```python
from build123d import *

# Parameters (mm, degrees)
SKETCH1_W                        = 170
SKETCH1_H                        = 150
BOSS_EXTRUDE1_DEPTH              = 5
FILLET1_R                        = 10
BOSS_EXTRUDE2_DEPTH              = 38
SKETCH29_W                       = 43
SKETCH29_H                       = 5
BOSS_EXTRUDE3_DEPTH              = 19
CUT_EXTRUDE1_START               = -2.9
SKETCH6_R                        = 16.5
CUT_EXTRUDE1_DEPTH               = 93.9
SKETCH13_R                       = 5.1
CUT_EXTRUDE2_DEPTH               = 4.7
TAP_DRILL_FOR_M2_TAP1_AT_2_COUNT = 2
TAP_DRILL_FOR_M2_TAP1_AT_2_PITCH = 8.5
TAP_DRILL_FOR_M2_TAP1_AT_3_COUNT = 2
TAP_DRILL_FOR_M2_TAP1_AT_3_PITCH = 14.722431864
TAP_DRILL_FOR_M2_TAP1_AT_4_COUNT = 2
TAP_DRILL_FOR_M2_TAP1_AT_4_PITCH = 14.722431864
FILLET2_R                        = 5
SKETCH28_W                       = 33
SKETCH28_H                       = 20
CUT_EXTRUDE3_DEPTH               = 10
MIRROR25_COPY_4_DEPTH            = 38
MIRROR25_START                   = -2.9
MIRROR25_COPY_5_SKETCH_R         = 16.5
MIRROR25_COPY_5_DEPTH            = 93.9
MIRROR25_COPY_6_SKETCH_R         = 5.1
MIRROR25_COPY_6_DEPTH            = 4.7
MIRROR25_COPY_11_SKETCH_W        = 33
MIRROR25_COPY_11_SKETCH_H        = 20
MIRROR25_COPY_11_DEPTH           = 10
FILLET4_R                        = 5
SKETCH33_W                       = 5
SKETCH33_H                       = 5.425553346
CUT_EXTRUDE4_DEPTH               = 10
CUT_EXTRUDE5_START               = -11
SKETCH34_W                       = 5
SKETCH34_H                       = 5
CUT_EXTRUDE5_DEPTH               = 28
MIRROR29_COPY_1_SKETCH_W         = 43
MIRROR29_COPY_1_SKETCH_H         = 5
MIRROR29_COPY_1_DEPTH            = 19
MIRROR29_START                   = -2.9
MIRROR29_COPY_2_SKETCH_R         = 16.5
MIRROR29_COPY_2_DEPTH            = 93.9
MIRROR29_COPY_3_SKETCH_W         = 5
MIRROR29_COPY_3_SKETCH_H         = 5.425553346
MIRROR29_COPY_3_DEPTH            = 10
MIRROR29_START_2                 = -11
MIRROR29_COPY_4_SKETCH_W         = 5
MIRROR29_COPY_4_SKETCH_H         = 5
MIRROR29_COPY_4_DEPTH            = 28


with BuildPart() as part:
    # Sketch1 → Boss-Extrude1 (new body)
    with BuildSketch(Plane(origin=(0, 0, 0), x_dir=(1, 0, 0), z_dir=(0, 1, 0))):
        Rectangle(SKETCH1_W, SKETCH1_H)
    extrude(amount=BOSS_EXTRUDE1_DEPTH)

    # Fillet1
    fillet1_edges = [part.edges().sort_by_distance(p)[0] for p in [
        (85, 2.5, 75),
        (-85, 2.5, 75),
        (-85, 2.5, -75),
        (85, 2.5, -75),
    ]]
    fillet(fillet1_edges, radius=FILLET1_R)

    # Sketch3 → Boss-Extrude2 (add)
    with BuildSketch(Plane.XZ):
        Polygon((-75, 75), (-75, 60), (-70, 60), (-70, 70), (-37, 70), (-37, 60), (-32, 60), (-32, 75), align=None)
    boss_extrude2 = extrude(amount=BOSS_EXTRUDE2_DEPTH)

    # Sketch29 → Boss-Extrude3 (add)
    with BuildSketch(Plane.XZ):
        with Locations((-53.5, 36.727703087)):
            Rectangle(SKETCH29_W, SKETCH29_H)
    boss_extrude3 = extrude(amount=BOSS_EXTRUDE3_DEPTH)

    # Sketch6 → Cut-Extrude1 (cut)
    with BuildSketch(Plane(origin=(0, 0, 70), x_dir=(-1, 0, 0), z_dir=(0, 0, -1)).offset(CUT_EXTRUDE1_START)):
        with Locations((53.5, -19)):
            Circle(SKETCH6_R)
    cut_extrude1 = extrude(amount=CUT_EXTRUDE1_DEPTH, mode=Mode.SUBTRACT)

    # Sketch13 → Cut-Extrude2 (cut)
    with BuildSketch(Plane(origin=(0, 0, 72.9), x_dir=(-1, 0, 0), z_dir=(0, 0, -1))):
        with Locations((53.5, -19)):
            Circle(SKETCH13_R)
    cut_extrude2 = extrude(amount=-CUT_EXTRUDE2_DEPTH, mode=Mode.SUBTRACT)

    # Sketch16 → Tap Drill for M2 Tap1 (revolve, cut)
    with BuildSketch(Plane(origin=(-46.138784068, -23.25, 72.9), x_dir=(0, 1, 0), z_dir=(1, 0, 0))):
        Polygon((0, 0), (0, 4.080688495), (0.8, 3.6), (0.8, 0), align=None)
    tap_drill_for_m2_tap1 = revolve(axis=Axis((-46.138784068, -23.25, 66.55), (0, 0, 1)), mode=Mode.SUBTRACT)

    # Tap Drill for M2 Tap1 at 2: Tap Drill for M2 Tap1 ×2
    with Locations(*[Vector(-0.86602540378444, -0.49999999999999756, 0) * (i * TAP_DRILL_FOR_M2_TAP1_AT_2_PITCH) for i in range(1, TAP_DRILL_FOR_M2_TAP1_AT_2_COUNT)]):
        add(tap_drill_for_m2_tap1, mode=Mode.SUBTRACT)

    # Tap Drill for M2 Tap1 at 3: Tap Drill for M2 Tap1 ×2
    with Locations(*[(-i * TAP_DRILL_FOR_M2_TAP1_AT_3_PITCH, 0, 0) for i in range(1, TAP_DRILL_FOR_M2_TAP1_AT_3_COUNT)]):
        add(tap_drill_for_m2_tap1, mode=Mode.SUBTRACT)

    # Tap Drill for M2 Tap1 at 4: Tap Drill for M2 Tap1 ×2
    with Locations(*[Vector(-0.49999999999999784, 0.8660254037844399, 0) * (i * TAP_DRILL_FOR_M2_TAP1_AT_4_PITCH) for i in range(1, TAP_DRILL_FOR_M2_TAP1_AT_4_COUNT)]):
        add(tap_drill_for_m2_tap1, mode=Mode.SUBTRACT)

    # Fillet2
    fillet2_edges = [part.edges().sort_by_distance(p)[0] for p in [
        (-32, -19, 75),
        (-75, -19, 75),
    ]]
    fillet(fillet2_edges, radius=FILLET2_R)

    # Sketch28 → Cut-Extrude3 (cut)
    with BuildSketch(Plane.XZ):
        with Locations((-53.5, 16.617641144)):
            Rectangle(SKETCH28_W, SKETCH28_H)
    cut_extrude3 = extrude(amount=-CUT_EXTRUDE3_DEPTH, mode=Mode.SUBTRACT)

    # Mirror14: Boss-Extrude2 across plane
    add(boss_extrude2.mirror(Plane.XY))

    # Mirror15: Cut-Extrude1, Cut-Extrude2 across plane
    add(cut_extrude1.mirror(Plane.XY), mode=Mode.SUBTRACT)
    add(cut_extrude2.mirror(Plane.XY), mode=Mode.SUBTRACT)

    # Mirror16: Tap Drill for M2 Tap1 across plane
    add(tap_drill_for_m2_tap1.mirror(Plane.XY), mode=Mode.SUBTRACT)

    # Mirror16 copy 1 sketch → Mirror16 copy 1 (revolve, cut)
    with BuildSketch(Plane(origin=(-53.5, -27.5, -72.9), x_dir=(0, 1, 0), z_dir=(1, 0, 0))):
        Polygon((0, 0), (0, -4.080688495), (0.8, -3.6), (0.8, 0), align=None)
    revolve(axis=Axis((-53.5, -27.5, -66.55), (0, 0, 1)), mode=Mode.SUBTRACT)

    # Mirror16 copy 2 sketch → Mirror16 copy 2 (revolve, cut)
    with BuildSketch(Plane(origin=(-60.861215932, -23.25, -72.9), x_dir=(0, 1, 0), z_dir=(1, 0, 0))):
        Polygon((0, 0), (0, -4.080688495), (0.8, -3.6), (0.8, 0), align=None)
    revolve(axis=Axis((-60.861215932, -23.25, -66.55), (0, 0, 1)), mode=Mode.SUBTRACT)

    # Mirror16 copy 3 sketch → Mirror16 copy 3 (revolve, cut)
    with BuildSketch(Plane(origin=(-53.5, -10.5, -72.9), x_dir=(0, 1, 0), z_dir=(1, 0, 0))):
        Polygon((0, 0), (0, -4.080688495), (0.8, -3.6), (0.8, 0), align=None)
    revolve(axis=Axis((-53.5, -10.5, -66.55), (0, 0, 1)), mode=Mode.SUBTRACT)

    # Mirror24: Cut-Extrude3 across plane
    add(cut_extrude3.mirror(Plane.XY), mode=Mode.SUBTRACT)

    # Mirror25: Boss-Extrude2, Cut-Extrude1, Cut-Extrude2, Tap Drill for M2 Tap1, Cut-Extrude3 across plane
    add(boss_extrude2.mirror(Plane(origin=(0, 0, 0), x_dir=(0, 0, 1), z_dir=(1, 0, 0))))
    add(cut_extrude1.mirror(Plane(origin=(0, 0, 0), x_dir=(0, 0, 1), z_dir=(1, 0, 0))), mode=Mode.SUBTRACT)
    add(cut_extrude2.mirror(Plane(origin=(0, 0, 0), x_dir=(0, 0, 1), z_dir=(1, 0, 0))), mode=Mode.SUBTRACT)
    add(tap_drill_for_m2_tap1.mirror(Plane(origin=(0, 0, 0), x_dir=(0, 0, 1), z_dir=(1, 0, 0))), mode=Mode.SUBTRACT)
    add(cut_extrude3.mirror(Plane(origin=(0, 0, 0), x_dir=(0, 0, 1), z_dir=(1, 0, 0))), mode=Mode.SUBTRACT)

    # Mirror25 copy 1 sketch → Mirror25 copy 1 (revolve, cut)
    with BuildSketch(Plane(origin=(53.5, -27.5, 72.9), x_dir=(0, 1, 0), z_dir=(-1, 0, 0))):
        Polygon((0, 0), (0, -4.080688495), (0.8, -3.6), (0.8, 0), align=None)
    revolve(axis=Axis((53.5, -27.5, 66.55), (0, 0, -1)), mode=Mode.SUBTRACT)

    # Mirror25 copy 2 sketch → Mirror25 copy 2 (revolve, cut)
    with BuildSketch(Plane(origin=(60.861215932, -23.25, 72.9), x_dir=(0, 1, 0), z_dir=(-1, 0, 0))):
        Polygon((0, 0), (0, -4.080688495), (0.8, -3.6), (0.8, 0), align=None)
    revolve(axis=Axis((60.861215932, -23.25, 66.55), (0, 0, -1)), mode=Mode.SUBTRACT)

    # Mirror25 copy 3 sketch → Mirror25 copy 3 (revolve, cut)
    with BuildSketch(Plane(origin=(53.5, -10.5, 72.9), x_dir=(0, 1, 0), z_dir=(-1, 0, 0))):
        Polygon((0, 0), (0, -4.080688495), (0.8, -3.6), (0.8, 0), align=None)
    revolve(axis=Axis((53.5, -10.5, 66.55), (0, 0, -1)), mode=Mode.SUBTRACT)

    # Mirror25 copy 4 sketch → Mirror25 copy 4 (add)
    with BuildSketch(Plane(origin=(0, 0, 0), x_dir=(-1, 0, 0), z_dir=(0, -1, 0))):
        Polygon((-75, 75), (-75, 60), (-70, 60), (-70, 70), (-37, 70), (-37, 60), (-32, 60), (-32, 75), align=None)
    extrude(amount=MIRROR25_COPY_4_DEPTH)

    # Mirror25 copy 5 sketch → Mirror25 copy 5 (cut)
    with BuildSketch(Plane.XY.offset(-70).offset(MIRROR25_START)):
        with Locations((53.5, -19)):
            Circle(MIRROR25_COPY_5_SKETCH_R)
    extrude(amount=MIRROR25_COPY_5_DEPTH, mode=Mode.SUBTRACT)

    # Mirror25 copy 6 sketch → Mirror25 copy 6 (cut)
    with BuildSketch(Plane.XY.offset(-72.9)):
        with Locations((53.5, -19)):
            Circle(MIRROR25_COPY_6_SKETCH_R)
    extrude(amount=-MIRROR25_COPY_6_DEPTH, mode=Mode.SUBTRACT)

    # Mirror25 copy 7 sketch → Mirror25 copy 7 (revolve, cut)
    with BuildSketch(Plane(origin=(46.138784068, -23.25, -72.9), x_dir=(0, 1, 0), z_dir=(-1, 0, 0))):
        Polygon((0, 0), (0, 4.080688495), (0.8, 3.6), (0.8, 0), align=None)
    revolve(axis=Axis((46.138784068, -23.25, -66.55), (0, 0, -1)), mode=Mode.SUBTRACT)

    # Mirror25 copy 8 sketch → Mirror25 copy 8 (revolve, cut)
    with BuildSketch(Plane(origin=(53.5, -27.5, -72.9), x_dir=(0, 1, 0), z_dir=(-1, 0, 0))):
        Polygon((0, 0), (0, 4.080688495), (0.8, 3.6), (0.8, 0), align=None)
    revolve(axis=Axis((53.5, -27.5, -66.55), (0, 0, -1)), mode=Mode.SUBTRACT)

    # Mirror25 copy 9 sketch → Mirror25 copy 9 (revolve, cut)
    with BuildSketch(Plane(origin=(60.861215932, -23.25, -72.9), x_dir=(0, 1, 0), z_dir=(-1, 0, 0))):
        Polygon((0, 0), (0, 4.080688495), (0.8, 3.6), (0.8, 0), align=None)
    revolve(axis=Axis((60.861215932, -23.25, -66.55), (0, 0, -1)), mode=Mode.SUBTRACT)

    # Mirror25 copy 10 sketch → Mirror25 copy 10 (revolve, cut)
    with BuildSketch(Plane(origin=(53.5, -10.5, -72.9), x_dir=(0, 1, 0), z_dir=(-1, 0, 0))):
        Polygon((0, 0), (0, 4.080688495), (0.8, 3.6), (0.8, 0), align=None)
    revolve(axis=Axis((53.5, -10.5, -66.55), (0, 0, -1)), mode=Mode.SUBTRACT)

    # Mirror25 copy 11 sketch → Mirror25 copy 11 (cut)
    with BuildSketch(Plane(origin=(0, 0, 0), x_dir=(-1, 0, 0), z_dir=(0, -1, 0))):
        with Locations((-53.5, 16.617641144)):
            Rectangle(MIRROR25_COPY_11_SKETCH_W, MIRROR25_COPY_11_SKETCH_H)
    extrude(amount=-MIRROR25_COPY_11_DEPTH, mode=Mode.SUBTRACT)

    # Fillet4
    fillet4_edges = [part.edges().sort_by_distance(p)[0] for p in [
        (-75, -19, -75),
        (-32, -19, -75),
        (32, -19, -75),
        (75, -19, -75),
        (75, -19, 75),
        (32, -19, 75),
    ]]
    fillet(fillet4_edges, radius=FILLET4_R)

    # Sketch33 → Cut-Extrude4 (cut)
    with BuildSketch(Plane.XZ):
        with Locations((-26.5, 36.94047976)):
            Rectangle(SKETCH33_W, SKETCH33_H)
    cut_extrude4 = extrude(amount=-CUT_EXTRUDE4_DEPTH, mode=Mode.SUBTRACT)

    # Sketch34 → Cut-Extrude5 (cut)
    with BuildSketch(Plane(origin=(0, 5, 0), x_dir=(1, 0, 0), z_dir=(0, 1, 0)).offset(CUT_EXTRUDE5_START)):
        with Locations((-80.5, -36.727703087)):
            Rectangle(SKETCH34_W, SKETCH34_H)
    cut_extrude5 = extrude(amount=CUT_EXTRUDE5_DEPTH, mode=Mode.SUBTRACT)

    # Mirror28: Boss-Extrude3, Cut-Extrude1, Cut-Extrude4, Cut-Extrude5 across plane
    add(boss_extrude3.mirror(Plane.XY))
    add(cut_extrude1.mirror(Plane.XY), mode=Mode.SUBTRACT)
    add(cut_extrude4.mirror(Plane.XY), mode=Mode.SUBTRACT)
    add(cut_extrude5.mirror(Plane.XY), mode=Mode.SUBTRACT)

    # Mirror29: Boss-Extrude3, Cut-Extrude1, Cut-Extrude4, Cut-Extrude5 across plane
    add(boss_extrude3.mirror(Plane(origin=(0, 0, 0), x_dir=(0, 0, 1), z_dir=(1, 0, 0))))
    add(cut_extrude1.mirror(Plane(origin=(0, 0, 0), x_dir=(0, 0, 1), z_dir=(1, 0, 0))), mode=Mode.SUBTRACT)
    add(cut_extrude4.mirror(Plane(origin=(0, 0, 0), x_dir=(0, 0, 1), z_dir=(1, 0, 0))), mode=Mode.SUBTRACT)
    add(cut_extrude5.mirror(Plane(origin=(0, 0, 0), x_dir=(0, 0, 1), z_dir=(1, 0, 0))), mode=Mode.SUBTRACT)

    # Mirror29 copy 1 sketch → Mirror29 copy 1 (add)
    with BuildSketch(Plane(origin=(0, 0, 0), x_dir=(-1, 0, 0), z_dir=(0, -1, 0))):
        with Locations((-53.5, 36.727703087)):
            Rectangle(MIRROR29_COPY_1_SKETCH_W, MIRROR29_COPY_1_SKETCH_H)
    extrude(amount=MIRROR29_COPY_1_DEPTH)

    # Mirror29 copy 2 sketch → Mirror29 copy 2 (cut)
    with BuildSketch(Plane.XY.offset(-70).offset(MIRROR29_START)):
        with Locations((53.5, -19)):
            Circle(MIRROR29_COPY_2_SKETCH_R)
    extrude(amount=MIRROR29_COPY_2_DEPTH, mode=Mode.SUBTRACT)

    # Mirror29 copy 3 sketch → Mirror29 copy 3 (cut)
    with BuildSketch(Plane(origin=(0, 0, 0), x_dir=(-1, 0, 0), z_dir=(0, -1, 0))):
        with Locations((-26.5, 36.94047976)):
            Rectangle(MIRROR29_COPY_3_SKETCH_W, MIRROR29_COPY_3_SKETCH_H)
    extrude(amount=-MIRROR29_COPY_3_DEPTH, mode=Mode.SUBTRACT)

    # Mirror29 copy 4 sketch → Mirror29 copy 4 (cut)
    with BuildSketch(Plane(origin=(0, 5, 0), x_dir=(-1, 0, 0), z_dir=(0, 1, 0)).offset(MIRROR29_START_2)):
        with Locations((-80.5, -36.727703087)):
            Rectangle(MIRROR29_COPY_4_SKETCH_W, MIRROR29_COPY_4_SKETCH_H)
    extrude(amount=MIRROR29_COPY_4_DEPTH, mode=Mode.SUBTRACT)


solid = part.part
```
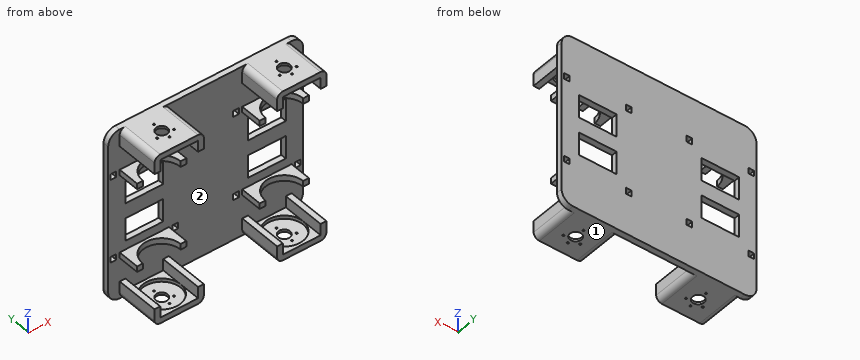
Could you check a few things on this model? Use its own coordinates, in mm. Face numbers are marked on the shaded views. Coordinates: 2 decimals unless noted, no trailing zeros. Write each loop counter-clockwise with the first axis right and the second up, starting at its lowest first coordinate (ties: lowest second). Pieces come first, ordered by that corner, then holes. Notation, with made-up numbers: (28, 1.25) -> (72, 1.25) arc R23 cw to (72, 28.25) -> close; hole circle Ø8 at (33, 47). An arc over 180 degrees is marked (long way). One line per question, with ' | ' between items. Start each with the question number.
1. Will these pins go through, and if not, where does the flat tip stop? P1, Ø10, axis at x = 14, z = 11, coming from the -Y side; P2, Ø1.4, axis at x = 46.14, y = -23.25, coming from the -Z side; P3, Ø3, axis at y = -22.5, z = -64.5, coming from the -X side; P4, Ø13.5, axis at x = -53.5, y = -19, coming from the -Z side.
2. If we section it at C-C (y = -32.5): Count the separate pieces of the cut face and the enclosed holes in it, and give its area (3 significant figures).
3. Please list where these lines run through material, in increasing order: line 1 along Z through (x, y) = (-42.5, 2); line 2 along X through (y, z) = (-11, 68); line 3 along X through (y, z) = (-19, -72.05).
4. Thinking about a two-plate mould opening in X: for the marked faces 1 and 2, which applies, pulls with the +X half, pulls with the -X half, needs draft (parallel to the pull), parting line crosses it, or undercut?
5. If we section it at D-D (z = 54): Please give me the cut outline in (x, y).
6. If we section it at B-B (x = 35): Please give me the cut outline in (y, z).
7. If we section it at A-A (z = -22.5): Please give me the cut outline in (x, y).
Return value:
1) P1: stops at y = 0 | P2: passes through | P3: stops at x = -75 | P4: stops at z = -75
2) separate pieces: 4 | enclosed holes: 0 | area: 997 mm²
3) line 1: z = -75 to -26.62, -6.62 to 6.62, 26.62 to 75 | line 2: x = -75 to -70, -37 to -32, 32 to 37, 70 to 75 | line 3: x = -74.56 to -70, -37 to -32.44, 32.44 to 37, 70 to 74.56
4) face 1: needs draft | face 2: undercut
5) outline: (-85, 0) -> (85, 0) -> (85, 5) -> (-85, 5) -> close
6) outline: (-38, -74.58) -> (0, -74.58) -> (0, -75) -> (5, -75) -> (5, 75) -> (0, 75) -> (0, 74.58) -> (-38, 74.58) -> (-38, 60) -> (0, 60) -> (0, 39.23) -> (-19, 39.23) -> (-19, 34.23) -> (0, 34.23) -> (0, -34.23) -> (-19, -34.23) -> (-19, -39.23) -> (0, -39.23) -> (0, -60) -> (-38, -60) -> close
7) outline: (-85, 0) -> (-70, 0) -> (-70, 5) -> (-85, 5) -> close; (-37, 0) -> (37, 0) -> (37, 5) -> (-37, 5) -> close; (70, 0) -> (85, 0) -> (85, 5) -> (70, 5) -> close
